from build123d import *

# Parameters (mm, degrees)
SKETCH1_W           = 500
SKETCH1_H           = 320
SKETCH1_W_2         = 480
SKETCH1_H_2         = 300
BOSS_EXTRUDE1_DEPTH = 20
SKETCH2_R           = 3
CUT_EXTRUDE1_DEPTH  = 500
SKETCH3_R           = 3
CUT_EXTRUDE2_DEPTH  = 320


with BuildPart() as part:
    # Sketch1 → Boss-Extrude1 (new body)
    with BuildSketch(Plane(origin=(0, 0, 0), x_dir=(1, 0, 0), z_dir=(0, 1, 0))):
        Rectangle(SKETCH1_W, SKETCH1_H)
        Rectangle(SKETCH1_W_2, SKETCH1_H_2, mode=Mode.SUBTRACT)
    extrude(amount=BOSS_EXTRUDE1_DEPTH)

    # Sketch2 → Cut-Extrude1 (cut)
    with BuildSketch(Plane(origin=(250, 0, 0), x_dir=(0, 0, -1), z_dir=(1, 0, 0))):
        with Locations((75, 10)):
            Circle(SKETCH2_R)
        with Locations((-75, 10)):
            Circle(SKETCH2_R)
    extrude(amount=-CUT_EXTRUDE1_DEPTH, mode=Mode.SUBTRACT)

    # Sketch3 → Cut-Extrude2 (cut)
    with BuildSketch(Plane.XY.offset(160)):
        with Locations((-180, 10)):
            Circle(SKETCH3_R)
        with Locations((180, 10)):
            Circle(SKETCH3_R)
    extrude(amount=-CUT_EXTRUDE2_DEPTH, mode=Mode.SUBTRACT)


solid = part.part
Can you work these out from the model? Positions are in its coordinate system, mm. A direction names the side the tool comes from. Give positions to 0.01 mm unless a question says otherwise; leave off trailing zeros. Order: outer loops, then holes, each group sorted by start corner. A loop starts at its lowest first (then second) coordinate and runs counter-clockwise, first axis right, second up. Notation, with made-up numbers: M 58,26 L 70,26 A6 cw 70,32 Z; hole C 5.25,-20 d5. An arc over 180 degrees is marked long. Use one line per item in the form item = value.
Item 1: If we section it at C-C, the plane y = 3.5: Write out the boundary of the cut face in (x, z).
Values follow:
outline = M -250,-160 L 250,-160 L 250,160 L -250,160 Z; hole M -240,-150 L 240,-150 L 240,150 L -240,150 Z
Item 2: If we section it at A-A, the plane z = -18: Write out the boundary of the cut face in (x, y).
Values follow:
outline = M -250,0 L -240,0 L -240,20 L -250,20 Z; M 240,0 L 250,0 L 250,20 L 240,20 Z
Item 3: Thinking about a two-plate mould opening in X: for faces 1 (the flat face through (-3, 10, -160)), 2 (the flat face through (240, 10, 2)), 3 (the flat face through (-250, 10, 2)), which applies, pulls with the +X half, pulls with the -X half, needs draft (parallel to the pull), parting line crosses it, or undercut?
Values follow:
face_1 = needs draft
face_2 = undercut
face_3 = pulls with the -X half
Item 4: If I drill on line 1 along X through (y, z) = (9, 64); line 2 along Z through (x, y) = (-132, 1); line 3 along Y through (x, z) = (-245.75, -75), over which ranges is the centre line in solid material (lowest first)? Write a range as [from, to].
Values follow:
line_1 = [-250, -240], [240, 250]
line_2 = [-160, -150], [150, 160]
line_3 = [0, 7], [13, 20]
Item 5: For faces 4 (the flat face through (-240, 10, 2)), 5 (the flat face through (-3, 10, 160)), which set-ups out of +Z, -Z, +X, -X, +Y, -Y let a thin tool reach every point of the face, with its end or its side?
Values follow:
face_4 = +Y, -Y
face_5 = +Z, +X, -X, +Y, -Y
Item 6: Will this pin go through, and if not, where does the flat tip stop? pin 1 Ø9.5 at (x, y) = (-180, 10) entering from +Z.
Values follow:
pin_1 = 160
Item 7: If we section it at B-B, the plane x = -77.5: Write out the boundary of the cut face in (y, z).
Values follow:
outline = M 0,-160 L 20,-160 L 20,-150 L 0,-150 Z; M 0,150 L 20,150 L 20,160 L 0,160 Z
